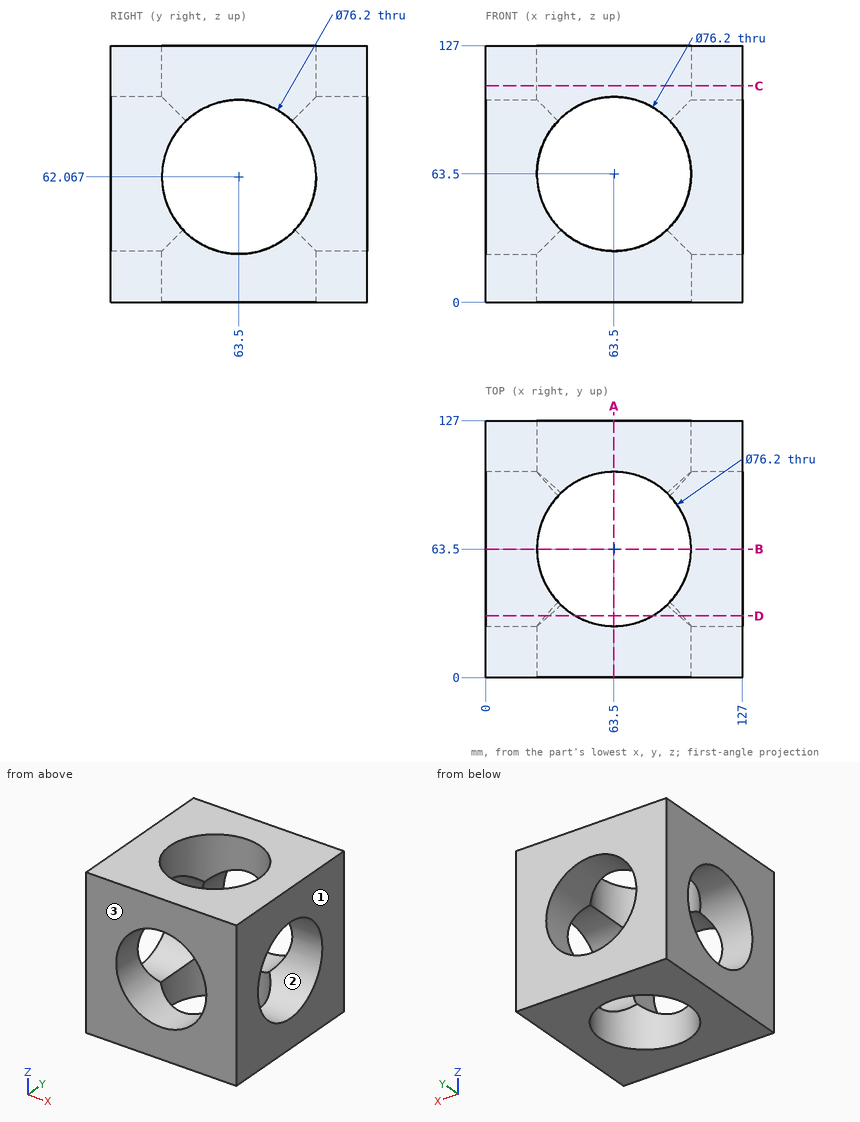
Could you check a few things on this drawing? It's one solid part, dimensions in mm from its lowest x, y, z. Coordinates: 2 decimals unless noted, no trailing zeros. Loops run counter-clockwise (first coordinate to the right, second up) from the corner with the lowest first, then second, coordinate; pieces in that order, holes last. Notation, with made-up numbers: (73.5, -9) - (124.5, -9) arc R10 ccw to (124.5, -2) - close; hole circle Ø7 at (-29.75, 55.5). An arc over 180 degrees is marked (long way). Answer as a JSON object with one key per item and string values. Group by question number.
Item 1: For pin 1 (1 mm diameter, centred on x = 105, y = 52, fed in from -Z), with a flat end and sliding along its axis, tell me the tip position at first contact or that it passes through.
Item 2: If we section it at A-A (x = 63.5): List the corners of the cut face in (y, z) for me.
Item 3: If I drill on L1, parallel to Y at x = 63, z = 14; L2, parallel to Z at x = 17.5, y = 63.5, over which ranges is the centre line in solid material (lowest first)? Write a range as from..to.
Item 4: If we section it at C-C (z = 107): List the corners of the cut face in (x, y) for me, plus the area to 3 significant figures.
Item 5: If we section it at B-B (y = 63.5): List the corners of the cut face in (x, z) for me, plus the area to 3 significant figures.
Item 6: If we section it at D-D (y = 30.5): List the corners of the cut face in (x, z) for me.
Item 7: If we mould it in two halves opening along Y, with no side actions, what happens to the marked faces 1, 2 and 3? For each: released by +Y, released by -Y, zero draft, split by the parting line, or undercut.
Returned:
{
 "1": {"pin 1": "stops at z = 0"},
 "2": {"outline": "(0, 0) - (25.4, 0) - (25.4, 25.4) - (0, 25.4) - close; (0, 101.6) - (25.4, 101.6) - (25.4, 127) - (0, 127) - close; (101.6, 0) - (127, 0) - (127, 25.4) - (101.6, 25.4) - close; (101.6, 101.6) - (127, 101.6) - (127, 127) - (101.6, 127) - close"},
 "3": {"L1": "y = 0..25.4, 101.6..127", "L2": "z = 0..23.97, 100.17..127"},
 "4": {"outline": "(0, 0) - (127, 0) - (127, 127) - (0, 127) - close; hole circle Ø76.2 at (63.5, 63.5)", "area": "11,600 mm²"},
 "5": {"outline": "(0, 0) - (25.4, 0) - (25.4, 23.97) - (0, 23.97) - close; (0, 100.17) - (25.4, 100.17) - (25.4, 127) - (0, 127) - close; (101.6, 0) - (127, 0) - (127, 23.97) - (101.6, 23.97) - close; (101.6, 100.17) - (127, 100.17) - (127, 127) - (101.6, 127) - close", "area": "2,580 mm²"},
 "6": {"outline": "(0, 0) - (44.46, 0) - (44.46, 30.5) arc R38.1 cw to (31.37, 43.02) - (0, 43.02) - close; (0, 81.11) - (29.71, 81.11) arc R38.1 cw to (44.46, 96.5) - (44.46, 127) - (0, 127) - close; (82.54, 0) - (127, 0) - (127, 43.02) - (95.63, 43.02) arc R38.1 cw to (82.54, 30.5) - close; (82.54, 96.5) arc R38.1 cw to (97.29, 81.11) - (127, 81.11) - (127, 127) - (82.54, 127) - close"},
 "7": {"face 1": "zero draft", "face 2": "undercut", "face 3": "released by -Y"}
}
